Input: part model. Units: mm. Frame: model coordinates. Face numbers are marked on the shaded views. A direction names the side the tool comes from. Round coordinates to 2 decimals unless told otherwise and drop trailing zeros. Loops run counter-clockwise (first coordinate to the right, second up) from the corner with the lowest first, then second, coordinate; pieces in that order, holes last. Notation, with made-up numbers: M 29,34.25 L 72,34.25 A13 cw 72,56.25 Z; hole C 10,42 d5. An arc over 180 degrees is marked long. Return JSON: item names as keys, results as strings. Group by question number.
1) Section B-B (y = 7.5). Output: boundary loops of the cut face in (x, z), plus the area to 3 significant figures.
2) Access query for the marked faces 1 and 2. Directions: +Z, -Z, +X, -X, +Y, -Y. A direction counts if a zero-diameter tool reaches every point of the face in a straight line with its end or side. Return the directions, or none.
3) Section C-C (x = 50.5). Output: boundary loops of the cut face in (y, z).
4) Material intervals for line 1 (X direction, y = -28.5, z = 4); line 2 (Z direction, x = 182, y = -37); line 3 (Y direction, x = 108.5, z = -27), sorted ascending. Write a range as from..to.
5) Section A-A (y = -11). Output: boundary loops of the cut face in (x, z), plus the area to 3 significant figures.
6) Contact query for flat-ended pins moving along their axis: P1, Ø1.7, axis at x = 4.9, z = -12.7, coming from the -Y side; P2, Ø3.5, axis at x = 119.2, z = 25.4, coming from the +Y side; P3, Ø2.5, axis at x = 208.1, z = 12.7, coming from the +Y side. Output: stop coordinate, or through.
7) Mould query, pull axis X, two halves, no side actions, for the marked faces 3, 4, 5 and 6. Classes: +X half, -X half, draft (parallel to the pull), parting line (faces both ways), or undercut.
from build123d import *

# Parameters (mm, degrees)
SKETCH1_R           = 10
BOSS_EXTRUDE1_DEPTH = 6
SKETCH2_R           = 1.65
CUT_EXTRUDE1_DEPTH  = 16.362291496
SKETCH5_R           = 10
BOSS_EXTRUDE2_DEPTH = 6
SKETCH6_R           = 3.15
BOSS_EXTRUDE3_DEPTH = 6
BOSS_EXTRUDE4_REACH = 216.59
SKETCH7_W           = 80
SKETCH7_H           = 6
LOFT1_START         = 34
LOFT1_DEPTH         = 6
LOFT2_START         = -40
LOFT2_DEPTH         = 6
SKETCH10_R          = 1.45
CUT_EXTRUDE3_DEPTH  = 230.008733458
CUT_EXTRUDE4_REACH  = 222.384
SKETCH13_R          = 2.65
SKETCH13_R_2        = 1.65


# Read off the part's stored shape, not the designer's step: Loft1, Loft2
with BuildPart() as part:
    # Sketch1 → Boss-Extrude1 (new body)
    with BuildSketch(Plane(origin=(0, 0, 0), x_dir=(0, 0, -1), z_dir=(1, 0, 0))):
        Circle(SKETCH1_R)
    extrude(amount=BOSS_EXTRUDE1_DEPTH)

    # Sketch2 → Cut-Extrude1 (cut, through all)
    with BuildSketch(Plane(origin=(6, 0, 0), x_dir=(0, 0, -1), z_dir=(1, 0, 0))):
        Circle(SKETCH2_R)
    extrude(amount=-CUT_EXTRUDE1_DEPTH, mode=Mode.SUBTRACT)

    # Sketch5 → Boss-Extrude2 (add)
    with BuildSketch(Plane.ZY):
        with BuildLine():
            Line((-40, 0), (-40, -40))
            Line((-40, -40), (40, -40))
            Line((40, -40), (40, 0))
            ThreePointArc((40, 0), (0, 40), (-40, 0))
        make_face()
        Circle(SKETCH5_R, mode=Mode.SUBTRACT)
    extrude(amount=-BOSS_EXTRUDE2_DEPTH)


with BuildPart() as body_2:
    # Sketch6 → Boss-Extrude3 (new body)
    with BuildSketch(Plane(origin=(213, 0, 0), x_dir=(0, 0, -1), z_dir=(1, 0, 0))):
        with BuildLine():
            Line((-40, 0), (-40, -40))
            Line((-40, -40), (40, -40))
            Line((40, -40), (40, 0))
            ThreePointArc((40, 0), (0, 40), (-40, 0))
        make_face()
        Circle(SKETCH6_R, mode=Mode.SUBTRACT)
    extrude(amount=-BOSS_EXTRUDE3_DEPTH)

    # Sketch7 → Boss-Extrude4 (add, up to next)
    with BuildSketch(Plane(origin=(6, 0, 0), x_dir=(0, 0, -1), z_dir=(1, 0, 0)), mode=Mode.PRIVATE) as boss_extrude4_sk1:
        with Locations((0, -37)):
            Rectangle(SKETCH7_W, SKETCH7_H)
    boss_extrude4_tool1 = extrude(boss_extrude4_sk1.sketch, amount=BOSS_EXTRUDE4_REACH, mode=Mode.PRIVATE) - body_2.part

    add(part.part)  # Boss-Extrude4 merges part
    add(boss_extrude4_tool1.solids().sort_by_distance((6, -37, 0))[0])

    # Loft1 outline → Loft1 (add)
    with BuildSketch(Plane.XY.offset(LOFT1_START)):
        Polygon((6, -34), (26, -34), (6, -14), align=None)
    loft1 = extrude(amount=LOFT1_DEPTH)

    # Loft2 outline → Loft2 (add)
    with BuildSketch(Plane.XY.offset(LOFT2_START)):
        Polygon((6, -34), (26, -34), (6, -14), align=None)
    loft2 = extrude(amount=LOFT2_DEPTH)

    # Mirror1: Loft1, Loft2 across plane
    add(loft1.mirror(Plane(origin=(106.5, 0, 0), x_dir=(0, 0, 1), z_dir=(1, 0, 0))))
    add(loft2.mirror(Plane(origin=(106.5, 0, 0), x_dir=(0, 0, 1), z_dir=(1, 0, 0))))

    # Sketch10 → Cut-Extrude3 (cut, through all)
    with BuildSketch(Plane(origin=(0, -34, 0), x_dir=(1, 0, 0), z_dir=(0, 1, 0))):
        with Locations(Location((106.5, 0, 0), (0, 0, 270))):
            Circle(SKETCH10_R)
        with Locations(Location((93.8, 0, 0), (0, 0, 270))):
            Circle(SKETCH10_R)
        with Locations(Location((81.1, 0, 0), (0, 0, 270))):
            Circle(SKETCH10_R)
        with Locations(Location((68.4, 0, 0), (0, 0, 270))):
            Circle(SKETCH10_R)
        with Locations(Location((55.7, 0, 0), (0, 0, 270))):
            Circle(SKETCH10_R)
        with Locations(Location((43, 0, 0), (0, 0, 270))):
            Circle(SKETCH10_R)
        with Locations(Location((30.3, 0, 0), (0, 0, 270))):
            Circle(SKETCH10_R)
        with Locations(Location((17.6, 0, 0), (0, 0, 270))):
            Circle(SKETCH10_R)
        with Locations(Location((4.9, 0, 0), (0, 0, 270))):
            Circle(SKETCH10_R)
        with Locations(Location((119.2, 0, 0), (0, 0, 270))):
            Circle(SKETCH10_R)
        with Locations(Location((131.9, 0, 0), (0, 0, 270))):
            Circle(SKETCH10_R)
        with Locations(Location((144.6, 0, 0), (0, 0, 270))):
            Circle(SKETCH10_R)
        with Locations(Location((157.3, 0, 0), (0, 0, 270))):
            Circle(SKETCH10_R)
        with Locations(Location((170, 0, 0), (0, 0, 270))):
            Circle(SKETCH10_R)
        with Locations(Location((182.7, 0, 0), (0, 0, 270))):
            Circle(SKETCH10_R)
        with Locations(Location((195.4, 0, 0), (0, 0, 270))):
            Circle(SKETCH10_R)
        with Locations(Location((208.1, 0, 0), (0, 0, 270))):
            Circle(SKETCH10_R)
        with Locations(Location((106.5, 12.7, 0), (0, 0, 270))):
            Circle(SKETCH10_R)
        with Locations(Location((93.8, 12.7, 0), (0, 0, 270))):
            Circle(SKETCH10_R)
        with Locations(Location((81.1, 12.7, 0), (0, 0, 270))):
            Circle(SKETCH10_R)
        with Locations(Location((68.4, 12.7, 0), (0, 0, 270))):
            Circle(SKETCH10_R)
        with Locations(Location((55.7, 12.7, 0), (0, 0, 270))):
            Circle(SKETCH10_R)
        with Locations(Location((43, 12.7, 0), (0, 0, 270))):
            Circle(SKETCH10_R)
        with Locations(Location((30.3, 12.7, 0), (0, 0, 270))):
            Circle(SKETCH10_R)
        with Locations(Location((17.6, 12.7, 0), (0, 0, 270))):
            Circle(SKETCH10_R)
        with Locations(Location((4.9, 12.7, 0), (0, 0, 270))):
            Circle(SKETCH10_R)
        with Locations(Location((119.2, 12.7, 0), (0, 0, 270))):
            Circle(SKETCH10_R)
        with Locations(Location((131.9, 12.7, 0), (0, 0, 270))):
            Circle(SKETCH10_R)
        with Locations(Location((144.6, 12.7, 0), (0, 0, 270))):
            Circle(SKETCH10_R)
        with Locations(Location((157.3, 12.7, 0), (0, 0, 270))):
            Circle(SKETCH10_R)
        with Locations(Location((170, 12.7, 0), (0, 0, 270))):
            Circle(SKETCH10_R)
        with Locations(Location((182.7, 12.7, 0), (0, 0, 270))):
            Circle(SKETCH10_R)
        with Locations(Location((195.4, 12.7, 0), (0, 0, 270))):
            Circle(SKETCH10_R)
        with Locations(Location((208.1, 12.7, 0), (0, 0, 270))):
            Circle(SKETCH10_R)
        with Locations(Location((106.5, 25.4, 0), (0, 0, 270))):
            Circle(SKETCH10_R)
        with Locations(Location((93.8, 25.4, 0), (0, 0, 270))):
            Circle(SKETCH10_R)
        with Locations(Location((81.1, 25.4, 0), (0, 0, 270))):
            Circle(SKETCH10_R)
        with Locations(Location((68.4, 25.4, 0), (0, 0, 270))):
            Circle(SKETCH10_R)
        with Locations(Location((55.7, 25.4, 0), (0, 0, 270))):
            Circle(SKETCH10_R)
        with Locations(Location((43, 25.4, 0), (0, 0, 270))):
            Circle(SKETCH10_R)
        with Locations(Location((30.3, 25.4, 0), (0, 0, 270))):
            Circle(SKETCH10_R)
        with Locations(Location((17.6, 25.4, 0), (0, 0, 270))):
            Circle(SKETCH10_R)
        with Locations(Location((4.9, 25.4, 0), (0, 0, 270))):
            Circle(SKETCH10_R)
        with Locations(Location((119.2, 25.4, 0), (0, 0, 270))):
            Circle(SKETCH10_R)
        with Locations(Location((131.9, 25.4, 0), (0, 0, 270))):
            Circle(SKETCH10_R)
        with Locations(Location((144.6, 25.4, 0), (0, 0, 270))):
            Circle(SKETCH10_R)
        with Locations(Location((157.3, 25.4, 0), (0, 0, 270))):
            Circle(SKETCH10_R)
        with Locations(Location((170, 25.4, 0), (0, 0, 270))):
            Circle(SKETCH10_R)
        with Locations(Location((182.7, 25.4, 0), (0, 0, 270))):
            Circle(SKETCH10_R)
        with Locations(Location((195.4, 25.4, 0), (0, 0, 270))):
            Circle(SKETCH10_R)
        with Locations(Location((208.1, 25.4, 0), (0, 0, 270))):
            Circle(SKETCH10_R)
        with Locations(Location((106.5, -12.7, 0), (0, 0, 270))):
            Circle(SKETCH10_R)
        with Locations(Location((93.8, -12.7, 0), (0, 0, 270))):
            Circle(SKETCH10_R)
        with Locations(Location((81.1, -12.7, 0), (0, 0, 270))):
            Circle(SKETCH10_R)
        with Locations(Location((68.4, -12.7, 0), (0, 0, 270))):
            Circle(SKETCH10_R)
        with Locations(Location((55.7, -12.7, 0), (0, 0, 270))):
            Circle(SKETCH10_R)
        with Locations(Location((43, -12.7, 0), (0, 0, 270))):
            Circle(SKETCH10_R)
        with Locations(Location((30.3, -12.7, 0), (0, 0, 270))):
            Circle(SKETCH10_R)
        with Locations(Location((17.6, -12.7, 0), (0, 0, 270))):
            Circle(SKETCH10_R)
        with Locations(Location((4.9, -12.7, 0), (0, 0, 270))):
            Circle(SKETCH10_R)
        with Locations(Location((119.2, -12.7, 0), (0, 0, 270))):
            Circle(SKETCH10_R)
        with Locations(Location((131.9, -12.7, 0), (0, 0, 270))):
            Circle(SKETCH10_R)
        with Locations(Location((144.6, -12.7, 0), (0, 0, 270))):
            Circle(SKETCH10_R)
        with Locations(Location((157.3, -12.7, 0), (0, 0, 270))):
            Circle(SKETCH10_R)
        with Locations(Location((170, -12.7, 0), (0, 0, 270))):
            Circle(SKETCH10_R)
        with Locations(Location((182.7, -12.7, 0), (0, 0, 270))):
            Circle(SKETCH10_R)
        with Locations(Location((195.4, -12.7, 0), (0, 0, 270))):
            Circle(SKETCH10_R)
        with Locations(Location((208.1, -12.7, 0), (0, 0, 270))):
            Circle(SKETCH10_R)
        with Locations(Location((106.5, -25.4, 0), (0, 0, 270))):
            Circle(SKETCH10_R)
        with Locations(Location((93.8, -25.4, 0), (0, 0, 270))):
            Circle(SKETCH10_R)
        with Locations(Location((81.1, -25.4, 0), (0, 0, 270))):
            Circle(SKETCH10_R)
        with Locations(Location((68.4, -25.4, 0), (0, 0, 270))):
            Circle(SKETCH10_R)
        with Locations(Location((55.7, -25.4, 0), (0, 0, 270))):
            Circle(SKETCH10_R)
        with Locations(Location((43, -25.4, 0), (0, 0, 270))):
            Circle(SKETCH10_R)
        with Locations(Location((30.3, -25.4, 0), (0, 0, 270))):
            Circle(SKETCH10_R)
        with Locations(Location((17.6, -25.4, 0), (0, 0, 270))):
            Circle(SKETCH10_R)
        with Locations(Location((4.9, -25.4, 0), (0, 0, 270))):
            Circle(SKETCH10_R)
        with Locations(Location((119.2, -25.4, 0), (0, 0, 270))):
            Circle(SKETCH10_R)
        with Locations(Location((131.9, -25.4, 0), (0, 0, 270))):
            Circle(SKETCH10_R)
        with Locations(Location((144.6, -25.4, 0), (0, 0, 270))):
            Circle(SKETCH10_R)
        with Locations(Location((157.3, -25.4, 0), (0, 0, 270))):
            Circle(SKETCH10_R)
        with Locations(Location((170, -25.4, 0), (0, 0, 270))):
            Circle(SKETCH10_R)
        with Locations(Location((182.7, -25.4, 0), (0, 0, 270))):
            Circle(SKETCH10_R)
        with Locations(Location((195.4, -25.4, 0), (0, 0, 270))):
            Circle(SKETCH10_R)
        with Locations(Location((208.1, -25.4, 0), (0, 0, 270))):
            Circle(SKETCH10_R)
    extrude(amount=-CUT_EXTRUDE3_DEPTH, mode=Mode.SUBTRACT)

    # Sketch13 → Cut-Extrude4 (cut, up to next)
    with BuildSketch(Plane.ZY, mode=Mode.PRIVATE) as cut_extrude4_sk1:
        Circle(SKETCH13_R)
    cut_extrude4_tool1 = extrude(cut_extrude4_sk1.sketch, amount=-CUT_EXTRUDE4_REACH, mode=Mode.PRIVATE) & body_2.part
    # Sketch13 → Cut-Extrude4 (cut, up to next)
    with BuildSketch(Plane.ZY, mode=Mode.PRIVATE) as cut_extrude4_sk2:
        with Locations((-20, 20)):
            Circle(SKETCH13_R_2)
    cut_extrude4_tool2 = extrude(cut_extrude4_sk2.sketch, amount=-CUT_EXTRUDE4_REACH, mode=Mode.PRIVATE) & body_2.part
    # Sketch13 → Cut-Extrude4 (cut, up to next)
    with BuildSketch(Plane.ZY, mode=Mode.PRIVATE) as cut_extrude4_sk3:
        with Locations((-20, -20)):
            Circle(SKETCH13_R_2)
    cut_extrude4_tool3 = extrude(cut_extrude4_sk3.sketch, amount=-CUT_EXTRUDE4_REACH, mode=Mode.PRIVATE) & body_2.part
    # Sketch13 → Cut-Extrude4 (cut, up to next)
    with BuildSketch(Plane.ZY, mode=Mode.PRIVATE) as cut_extrude4_sk4:
        with Locations((20, -20)):
            Circle(SKETCH13_R_2)
    cut_extrude4_tool4 = extrude(cut_extrude4_sk4.sketch, amount=-CUT_EXTRUDE4_REACH, mode=Mode.PRIVATE) & body_2.part
    # Sketch13 → Cut-Extrude4 (cut, up to next)
    with BuildSketch(Plane.ZY, mode=Mode.PRIVATE) as cut_extrude4_sk5:
        with Locations((20, 20)):
            Circle(SKETCH13_R_2)
    cut_extrude4_tool5 = extrude(cut_extrude4_sk5.sketch, amount=-CUT_EXTRUDE4_REACH, mode=Mode.PRIVATE) & body_2.part
    add(cut_extrude4_tool1.solids().sort_by_distance((0, 0, 0))[0], mode=Mode.SUBTRACT)
    add(cut_extrude4_tool2.solids().sort_by_distance((0, 20, -20))[0], mode=Mode.SUBTRACT)
    add(cut_extrude4_tool3.solids().sort_by_distance((0, -20, -20))[0], mode=Mode.SUBTRACT)
    add(cut_extrude4_tool4.solids().sort_by_distance((0, -20, 20))[0], mode=Mode.SUBTRACT)
    add(cut_extrude4_tool5.solids().sort_by_distance((0, 20, 20))[0], mode=Mode.SUBTRACT)


solid = body_2.part
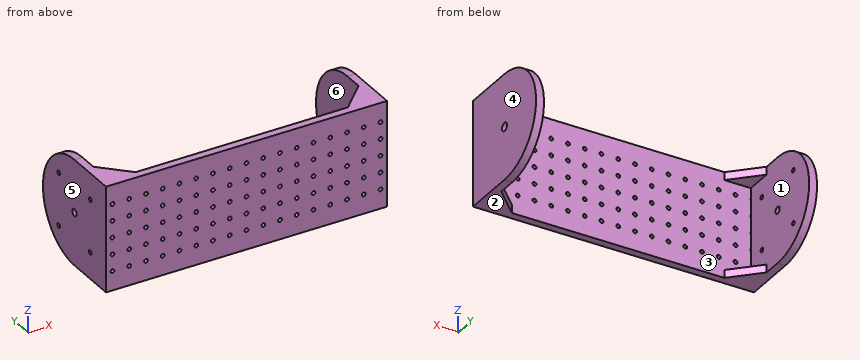
Returned:
{
 "1": {"outline": "M 0,-39.29 L 6,-39.29 L 6,39.29 L 0,39.29 Z; M 207,-39.29 L 213,-39.29 L 213,39.29 L 207,39.29 Z", "area": "943 mm^2"},
 "2": {"face 1": "+Y", "face 2": "-Z, +X, -X, +Y, -Y"},
 "3": {"outline": "M -40,-40 L -34,-40 L -34,40 L -40,40 Z"},
 "4": {"line 1": "x = 0..6, 207..213", "line 2": "z = -40..-26.67, -24.13..-13.97, -11.43..-1.27, 1.27..11.43, 13.97..24.13, 26.67..40", "line 3": "y = -40..-34"},
 "5": {"outline": "M 0,-40 L 6,-40 L 6,40 L 0,40 Z; M 207,-40 L 213,-40 L 213,40 L 207,40 Z", "area": "960 mm^2"},
 "6": {"P1": "stops at y = -34", "P2": "stops at y = -34", "P3": "stops at y = 38.33"},
 "7": {"face 3": "undercut", "face 4": "+X half", "face 5": "-X half", "face 6": "undercut"}
}
